```python
from build123d import *

# Parameters (mm, degrees)
ESBO_O3_W                = 16
ESBO_O3_H                = 16
RESSALTO_EXTRUS_O1_DEPTH = 12
ESBO_O4_R                = 3
RESSALTO_EXTRUS_O2_DEPTH = 6
RESSALTO_EXTRUS_O2_TAPER = 23


with BuildPart() as part:
    # Esboço1 → Revolução1 (revolve)
    with BuildSketch(Plane.XY, mode=Mode.PRIVATE) as revolu_o1_sk:
        Polygon((0, 47.333362218), (8, 47.333362218), (8, 43.391649695), (5.5, 43.391649695), (5.5, 37.391649695), (8, 37.391649695), (8, 33.514974639), (4, 33.514974639), (4, 30.514974639), (12.5, 30.514974639), (12.5, -1.485025361), (2, -1.485025361), (2, -2.985025361), (0, -2.985025361), align=None)
    revolve(revolu_o1_sk.sketch.rotate(Axis((0, 47.333362218, 0), (0, -1, 0)), 90), axis=Axis((0, 47.333362218, 0), (0, -1, 0)))

    # Esboço3 → Ressalto-extrusão1 (add)
    with BuildSketch(Plane.XZ.offset(2.985025361)):
        with Locations((0, 4)):
            Rectangle(ESBO_O3_W, ESBO_O3_H)
    extrude(amount=RESSALTO_EXTRUS_O1_DEPTH)

    # Esboço4 → Ressalto-extrusão2 (add)
    with BuildSketch(Plane.XZ.offset(14.985025361)):
        Circle(ESBO_O4_R)
    extrude(amount=RESSALTO_EXTRUS_O2_DEPTH, taper=RESSALTO_EXTRUS_O2_TAPER)


solid = part.part
```
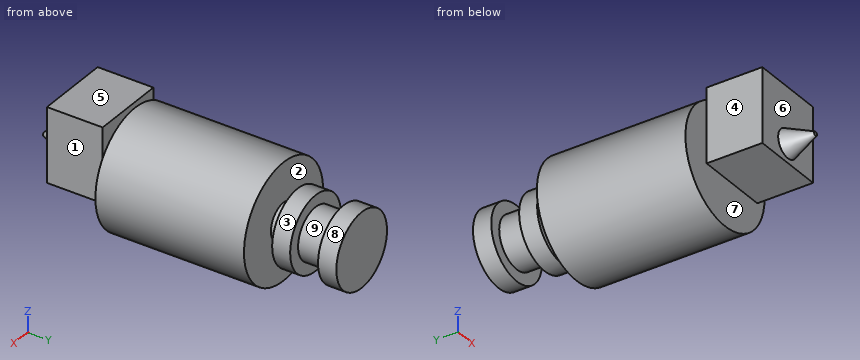
CAD build for the part. Positions are in the model's coordinates, mm. Face numbers are marked on the shaded views. A direction names the side the tool comes from. Round coordinates to 2 decimals unless told otherwise and drop trailing zeros. Write each loop counter-clockwise with the first axis right and the second up, starting at its lowest first coordinate (ties: lowest second). Pieces come first, ordered by that corner, then holes. Notation, with made-up numbers: M -4,-5 L 54,-5 A22 ccw 54,1 Z; hole C -33.75,32 d1. An arc over 180 degrees is marked long. One line per question, with ' | ' between items.
1. Pin check, flat tips, straight feed: pin 1 Ø1 at (x, z) = (-8.5, 5) entering from +Y (3 decimals); pin 2 Ø12 at (y, z) = (14, -3) entering from +X; pin 3 Ø13 at (x, z) = (-3, 7.5) entering from -Y; pin 4 Ø1 at (y, z) = (-3.5, 2) entering from +X. Stop position of each tip, or through.
Working result:
pin 1: y = 30.515 | pin 2: x = 12.5 | pin 3: y = -18.34 | pin 4: x = 8
2. Mould opens along Y. For the marked faces 6, 7, 8 and 9 say: pulls with the +Y half, pulls with the -Y half, needs draft (parallel to the pull), parting line crosses it, or undercut.
Working result:
face 6: pulls with the -Y half | face 7: undercut | face 8: needs draft | face 9: undercut
3. Cut at A-A on y = 0. Write the cut outline in (x, z), and give its area (3 significant figures).
Working result:
outline: C 0,0 d25 | area: 491 mm2
4. Which spindle directions (+Z, -Z, +X, -X, +Y, -Y) get a long thin tool onto all of the face, cutting with end or side? Do the marked faces 1, 2, 3, 4 and 5. Say none if no direction does.
Working result:
face 1: +Z, -Z, +X, -Y | face 2: none | face 3: +Y | face 4: +Z, -Z, -X, -Y | face 5: +Z, +X, -X, -Y
5. Cut at B-B on z = -11. Write the cut outline in (x, y), and give its area (3 significant figures).
Working result:
outline: M -5.94,-1.49 L 5.94,-1.49 L 5.94,30.51 L -5.94,30.51 Z | area: 380 mm2
6. Probe L1, parallel to Y at x = 2.75, z = 4.5; L2, parallel to Y at x = -0.75, z = -6; L3, parallel to Y at x = 5.5, z = -2.5. List the from-to ranges inside material, lowest first. Write a range as from..to.
Working result:
L1: -14.99..-2.99, -1.49..30.51, 33.51..47.33 | L2: -1.49..30.51, 33.51..37.39, 43.39..47.33 | L3: -14.99..-2.99, -1.49..30.51, 33.51..37.39, 43.39..47.33
7. Cut at C-C on y = -13. Write the cut outline in (x, z).
Working result:
outline: M -8,-4 L 8,-4 L 8,12 L -8,12 Z
